Could you check a few things on this model? Use its own coordinates, in mm. Give positions to 0.01 mm unless a question says otherwise; leave off trailing zeros. Order: outer loops, then holes, each group sorted by start corner. A loop starts at its lowest first (then second) coordinate and runs counter-clockwise, first axis right, second up. Notation, with made-up numbers: M 52.5,51.25 L 79.5,51.25 A25 ccw 79.5,88.25 Z; hole C 34.5,26 d2. An arc over 180 degrees is marked long. Use a Markdown table: item, result. Add a question column.
Item 1: Suppose I cut it at A-A on z = -93. Write out the boundary of the cut face in (x, y) (3 decimals).
Item 2: Suppose I cut it at C-C on y = 2.55. Count the separate pieces of the cut face and the enclosed holes in it, plus the area to 3 significant figures.
Item 3: I'm going to push flat-ended pins straight in: pin 1 Ø6.5 at (x, z) = (269.48, -153.19) entering from -Y; pin 2 Ø2 at (x, y) = (207, 2) entering from +Z. Where does each tip first touch, or does it pass through?
Item 4: If I drill on L1, parallel to X at y = 0.55, z = -98 (3 decimals); L2, parallel to X at y = 1.7, z = -154; L3, parallel to Z at x = 86.5, y = 1.5, over which ranges is the centre line in solid material (lowest first)? Write a range as from..to.
Item 5: Suppose I cut it at B-B on x = 111.5. Write out the boundary of the cut face in (y, z), plus the area to 3 significant figures.
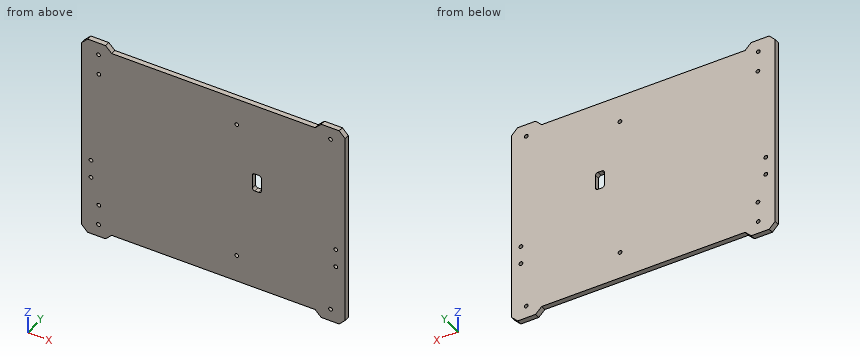
from build123d import *

# Parameters (mm, degrees)
SKETCH1_W                       = 279.4
SKETCH1_H                       = 215.9
BOSS_EXTRUDE1_DEPTH             = 5.5118
F_5_32_0_15625_DIAMETER_HOLE1_D = 3.96875
F_5_32_0_15625_DIAMETER_HOLE2_D = 3.96875
CUT_EXTRUDE2_DEPTH              = 6.5118
CHAMFER1_SIZE                   = 6.35
CUT_EXTRUDE3_DEPTH              = 6.5118


with BuildPart() as part:
    # Sketch1 → Boss-Extrude1 (new body)
    with BuildSketch(Plane(origin=(0, 0, 0), x_dir=(1, 0, 0), z_dir=(0, 1, 0))):
        with Locations((139.7, 107.95)):
            Rectangle(SKETCH1_W, SKETCH1_H)
    extrude(amount=BOSS_EXTRUDE1_DEPTH)

    # 5/32 (0.15625) Diameter Hole1 (through all)
    with Locations(Plane(origin=(0, 5.5118, 0), x_dir=(1, 0, 0), z_dir=(0, 1, 0))):
        with Locations((17.859375, 13.096875), (17.859375, 202.803125), (9.921875, 153.19375), (9.921875, 134.14375), (263.921875, 13.096875), (269.478125, 134.14375), (269.478125, 153.19375), (263.921875, 202.803125)):
            Hole(F_5_32_0_15625_DIAMETER_HOLE1_D / 2)

    # 5/32 (0.15625) Diameter Hole2 (through all)
    with Locations(Plane(origin=(0, 5.5118, 0), x_dir=(1, 0, 0), z_dir=(0, 1, 0))):
        with Locations((18.25625, 34.8361), (164.48405, 34.8361), (164.48405, 181.0639), (18.25625, 181.0639)):
            Hole(F_5_32_0_15625_DIAMETER_HOLE2_D / 2)

    # Sketch6 → Cut-Extrude2 (cut, through all)
    with BuildSketch(Plane(origin=(0, 5.5118, 0), x_dir=(1, 0, 0), z_dir=(0, 1, 0))):
        Polygon((247.65, 209.55), (254, 215.9), (25.4, 215.9), (31.75, 209.55), align=None)
        Polygon((25.4, 0), (254, 0), (247.65, 6.35), (31.75, 6.35), align=None)
    extrude(amount=-CUT_EXTRUDE2_DEPTH, mode=Mode.SUBTRACT)

    # Chamfer1
    chamfer1_edges = [part.edges().sort_by_distance(p)[0] for p in [
        (0, 2.7559, -215.9),
        (279.4, 2.7559, -215.9),
        (279.4, 2.7559, 0),
        (0, 2.7559, 0),
    ]]
    chamfer(chamfer1_edges, length=CHAMFER1_SIZE)

    # Sketch7 → Cut-Extrude3 (cut, through all)
    with BuildSketch(Plane(origin=(0, 5.5118, 0), x_dir=(1, 0, 0), z_dir=(0, 1, 0))):
        with BuildLine():
            Line((183.515, 101.6), (187.96, 101.6))
            ThreePointArc((187.96, 101.6), (189.756051224, 100.856051224), (190.5, 99.06))
            Line((190.5, 99.06), (190.5, 85.09))
            ThreePointArc((190.5, 85.09), (189.756051224, 83.293948776), (187.96, 82.55))
            Line((187.96, 82.55), (183.515, 82.55))
            ThreePointArc((183.515, 82.55), (181.718948776, 83.293948776), (180.975, 85.09))
            Line((180.975, 85.09), (180.975, 99.06))
            ThreePointArc((180.975, 99.06), (181.718948776, 100.856051224), (183.515, 101.6))
        make_face()
    extrude(amount=-CUT_EXTRUDE3_DEPTH, mode=Mode.SUBTRACT)


solid = part.part
Findings below:
| question | item | result |
|---|---|---|
| 1 | outline | M 0,0 L 180.975,0 L 180.975,5.512 L 0,5.512 Z; M 190.5,0 L 279.4,0 L 279.4,5.512 L 190.5,5.512 Z |
| 2 | separate pieces | 1 |
| 2 | enclosed holes | 13 |
| 2 | area | 57,100 mm^2 |
| 3 | pin 1 | stops at y = 0 |
| 3 | pin 2 | stops at z = -6.35 |
| 4 | L1 | x = 0..180.975, 190.5..279.4 |
| 4 | L2 | x = 0..8.11, 11.74..267.66, 271.29..279.4 |
| 4 | L3 | z = -209.55..-6.35 |
| 5 | outline | M 0,-209.55 L 5.51,-209.55 L 5.51,-6.35 L 0,-6.35 Z |
| 5 | area | 1,120 mm^2 |
